```python
from build123d import *

# Parameters (mm, degrees)
BOSS_EXTRUDE1_DEPTH        = 1.4
F_2_5_2_5_DIAMETER_SLOT1_D = 2.5
BOSS_EXTRUDE2_DEPTH        = 2
BOSS_EXTRUDE3_DEPTH        = 3
SKETCH8_W                  = 0.8
SKETCH8_H                  = 0.8
BOSS_EXTRUDE4_DEPTH        = 10


with BuildPart() as part:
    # Sketch1 → Boss-Extrude1 (new body)
    with BuildSketch(Plane.XY):
        Polygon((-17.623529412, 12), (-16.623529412, 13), (23.376470588, 13), (24.376470588, 12), (24.376470588, -10), (23.376470588, -11), (-17.623529412, -11), (-17.623529412, 0), (-16.823529412, 0), (-16.823529412, 5), (-17.623529412, 5), align=None)
    extrude(amount=BOSS_EXTRUDE1_DEPTH)

    # Ø2.5 (2.5) Diameter Slot1 (through all)
    with Locations(Plane.XY.offset(1.4)):
        with Locations((-15.874285672, -9.269193445), (-15.874285672, 11.312714255), (22.710754066, -9.269193445), (22.710754066, 11.312714255)):
            Hole(F_2_5_2_5_DIAMETER_SLOT1_D / 2)

    # Sketch6 → Boss-Extrude2 (add)
    with BuildSketch(Plane.XY.offset(1.4)):
        Polygon((-15.083529412, -6.7), (-0.083529412, -6.7), (-0.083529412, 8.3), (-14.083529412, 8.3), (-14.083529412, -1.2), (-15.083529412, -3.2), align=None)
    extrude(amount=BOSS_EXTRUDE2_DEPTH)

    # Sketch7 → Boss-Extrude3 (add)
    with BuildSketch(Plane.XY.offset(1.4)):
        with BuildLine():
            Line((22.126470588, 6.1), (22.126470588, 5.6))
            ThreePointArc((22.126470588, 5.6), (22.303247284, 5.526776695), (22.376470588, 5.35))
            Line((22.376470588, 5.35), (22.376470588, 3.78))
            ThreePointArc((22.376470588, 3.78), (22.303247284, 3.603223305), (22.126470588, 3.53))
            Line((22.126470588, 3.53), (22.126470588, 3.03))
            ThreePointArc((22.126470588, 3.03), (22.303247284, 2.956776695), (22.376470588, 2.78))
            Line((22.376470588, 2.78), (22.376470588, 1.21))
            ThreePointArc((22.376470588, 1.21), (22.303247284, 1.033223305), (22.126470588, 0.96))
            Line((22.126470588, 0.96), (22.126470588, 0.46))
            ThreePointArc((22.126470588, 0.46), (22.303247284, 0.386776695), (22.376470588, 0.21))
            Line((22.376470588, 0.21), (22.376470588, -1.36))
            ThreePointArc((22.376470588, -1.36), (22.303247284, -1.536776695), (22.126470588, -1.61))
            Line((22.126470588, -1.61), (22.126470588, -2.11))
            ThreePointArc((22.126470588, -2.11), (22.303247284, -2.183223305), (22.376470588, -2.36))
            Line((22.376470588, -2.36), (22.376470588, -3.93))
            ThreePointArc((22.376470588, -3.93), (22.303247284, -4.106776695), (22.126470588, -4.18))
            Line((22.126470588, -4.18), (22.126470588, -4.68))
            ThreePointArc((22.126470588, -4.68), (22.303247284, -4.753223305), (22.376470588, -4.93))
            Line((22.376470588, -4.93), (22.376470588, -6.75))
            ThreePointArc((22.376470588, -6.75), (22.303247284, -6.926776695), (22.126470588, -7))
            Line((22.126470588, -7), (19.626470588, -7))
            ThreePointArc((19.626470588, -7), (19.449693893, -6.926776695), (19.376470588, -6.75))
            Line((19.376470588, -6.75), (19.376470588, -4.93))
            ThreePointArc((19.376470588, -4.93), (19.449693893, -4.753223305), (19.626470588, -4.68))
            Line((19.626470588, -4.68), (19.626470588, -4.18))
            ThreePointArc((19.626470588, -4.18), (19.449693893, -4.106776695), (19.376470588, -3.93))
            Line((19.376470588, -3.93), (19.376470588, -2.36))
            ThreePointArc((19.376470588, -2.36), (19.449693893, -2.183223305), (19.626470588, -2.11))
            Line((19.626470588, -2.11), (19.626470588, -1.61))
            ThreePointArc((19.626470588, -1.61), (19.449693893, -1.536776695), (19.376470588, -1.36))
            Line((19.376470588, -1.36), (19.376470588, 0.21))
            ThreePointArc((19.376470588, 0.21), (19.449693893, 0.386776695), (19.626470588, 0.46))
            Line((19.626470588, 0.46), (19.626470588, 0.96))
            ThreePointArc((19.626470588, 0.96), (19.449693893, 1.033223305), (19.376470588, 1.21))
            Line((19.376470588, 1.21), (19.376470588, 2.78))
            ThreePointArc((19.376470588, 2.78), (19.449693893, 2.956776695), (19.626470588, 3.03))
            Line((19.626470588, 3.03), (19.626470588, 3.53))
            ThreePointArc((19.626470588, 3.53), (19.449693893, 3.603223305), (19.376470588, 3.78))
            Line((19.376470588, 3.78), (19.376470588, 5.35))
            ThreePointArc((19.376470588, 5.35), (19.449693893, 5.526776695), (19.626470588, 5.6))
            Line((19.626470588, 5.6), (19.626470588, 6.1))
            ThreePointArc((19.626470588, 6.1), (19.449693893, 6.173223305), (19.376470588, 6.35))
            Line((19.376470588, 6.35), (19.376470588, 8.17))
            ThreePointArc((19.376470588, 8.17), (19.449693893, 8.346776695), (19.626470588, 8.42))
            Line((19.626470588, 8.42), (22.126470588, 8.42))
            ThreePointArc((22.126470588, 8.42), (22.303247284, 8.346776695), (22.376470588, 8.17))
            Line((22.376470588, 8.17), (22.376470588, 6.35))
            ThreePointArc((22.376470588, 6.35), (22.303247284, 6.173223305), (22.126470588, 6.1))
        make_face()
    extrude(amount=BOSS_EXTRUDE3_DEPTH)

    # Sketch8 → Boss-Extrude4 (add)
    with BuildSketch(Plane.XY.offset(4.4)):
        with Locations((20.876470588, -5.84)):
            Rectangle(SKETCH8_W, SKETCH8_H)
        with Locations((20.876470588, -3.22)):
            Rectangle(SKETCH8_W, SKETCH8_H)
        with Locations((20.876470588, -0.6)):
            Rectangle(SKETCH8_W, SKETCH8_H)
        with Locations((20.876470588, 2.02)):
            Rectangle(SKETCH8_W, SKETCH8_H)
        with Locations((20.876470588, 4.64)):
            Rectangle(SKETCH8_W, SKETCH8_H)
        with Locations((20.876470588, 7.26)):
            Rectangle(SKETCH8_W, SKETCH8_H)
    extrude(amount=BOSS_EXTRUDE4_DEPTH)


solid = part.part
```
For this review, take the finished solid that the model builds, in its own axes (mm). A direction names the side the tool comes from. Coordinates: 2 decimals unless noted, no trailing zeros. Write each loop counter-clockwise with the first axis right and the second up, starting at its lowest first coordinate (ties: lowest second). Pieces come first, ordered by that corner, then holes. Notation, with made-up numbers: (30, -27) -> (49, -27) arc R18 ccw to (49, 8) -> close; hole circle Ø3 at (39, -31.5). An arc over 180 degrees is marked (long way). Put each result on its own line as item: value.
Q1. The part is to be moulded in two halves that separate along X. For faces 1 (the flat face through (-17, 0, 1)), 2 (the cylindrical face through (21.556, 10.834, 0.69)), 3 (the flat face through (-14.58, -2.19, 2.39)), say which applies: +X half, -X half, draft (parallel to the pull), parting line (faces both ways), or undercut.
From the geometry:
face 1: draft
face 2: undercut
face 3: -X half
Q2. Wall thickness on L1, parallel to Z at x = -13, y = -6; L2, parallel to Z at x = -12.5, y = 9.25; L3, parallel to X at y = 7, z = 10: over which ranges is each line inside the solid? List them lowest first.
From the geometry:
L1: z = 0 to 3.4
L2: z = 0 to 1.4
L3: x = 20.48 to 21.28
Q3. Take a section at D-D, the plane x = 2.5. State the section outline as (y, z) points, then the cut area to 3 significant figures.
From the geometry:
outline: (-11, 0) -> (13, 0) -> (13, 1.4) -> (-11, 1.4) -> close
area: 33.6 mm2
Q4. Take a section at B-B, the plane x = -9. State the section outline as (y, z) points, then the cut area to 3 significant figures.
From the geometry:
outline: (-11, 0) -> (13, 0) -> (13, 1.4) -> (8.3, 1.4) -> (8.3, 3.4) -> (-6.7, 3.4) -> (-6.7, 1.4) -> (-11, 1.4) -> close
area: 63.6 mm2
Q5. Tool access review of faces 4 (the flat face through (-8, -6.7, 2)), 5 (the flat face through (-15.084, -5, 2)), 6 (the flat face through (19.376, -6, 3)): name each direction out of +Z, -Z, +X, -X, +Y, -Y from which nothing blocks a thin tool from reaching the whole face with its end or side.
From the geometry:
face 4: +Z, -X, -Y
face 5: +Z, -X, +Y, -Y
face 6: +Z, +Y, -Y
Q6. Take a section at A-A, the plane z = 13.5. State the section outline as (x, y) points, then the cut area to 3 significant figures.
From the geometry:
outline: (20.48, -6.24) -> (21.28, -6.24) -> (21.28, -5.44) -> (20.48, -5.44) -> close; (20.48, -3.62) -> (21.28, -3.62) -> (21.28, -2.82) -> (20.48, -2.82) -> close; (20.48, -1) -> (21.28, -1) -> (21.28, -0.2) -> (20.48, -0.2) -> close; (20.48, 1.62) -> (21.28, 1.62) -> (21.28, 2.42) -> (20.48, 2.42) -> close; (20.48, 4.24) -> (21.28, 4.24) -> (21.28, 5.04) -> (20.48, 5.04) -> close; (20.48, 6.86) -> (21.28, 6.86) -> (21.28, 7.66) -> (20.48, 7.66) -> close
area: 3.84 mm2
Q7. Take a section at C-C, the plane y = -7.5. State the section outline as (x, z) points, then the cut area to 3 significant figures.
From the geometry:
outline: (-17.62, 0) -> (24.38, 0) -> (24.38, 1.4) -> (-17.62, 1.4) -> close
area: 58.8 mm2
Q8. Clearance check with flat-ended pins moving along their axes: pin 1 Ø1.5 at (x, y) = (7, 10) entering from +Z; pin 2 Ø1.5 at (y, z) = (7, 3.5) entering from -X; pin 3 Ø0.9 at (y, z) = (-3, 12) entering from -X; pin 4 Ø3 at (y, z) = (10, 3.5) entering from +X. State where each tip first meets the part, or that it passes through.
From the geometry:
pin 1: stops at z = 1.4
pin 2: stops at x = -14.08
pin 3: stops at x = 20.48
pin 4: passes through
